from build123d import *

# Parameters (mm, degrees)
EXTRUDE_1_DEPTH        = 6
HOLE_WIZARD_M6_1_D     = 5
HOLE_WIZARD_M6_1_DEPTH = 18
HOLE_WIZARD_M6_1_TIP   = 1.502151548
FILLET_1_R             = 10
HOLE_WIZARD_M10_1_D    = 8.5


with BuildPart() as part:
    # 草图1 → 凸台-拉伸1 (new body, symmetric)
    with BuildSketch(Plane.XY):
        Polygon((0, 0), (75, 0), (75, 15), (120, 15), (120, 40), (0, 40), align=None)
    extrude(amount=EXTRUDE_1_DEPTH, both=True)

    # M6 螺纹孔1
    with Locations(Plane(origin=(0, 0, 0), x_dir=(-1, 0, 0), z_dir=(0, -1, 0))):
        with Locations((-10, 0), (-65, 0)):
            Hole(HOLE_WIZARD_M6_1_D / 2, depth=HOLE_WIZARD_M6_1_DEPTH)
            with Locations((0, 0, -(HOLE_WIZARD_M6_1_DEPTH + HOLE_WIZARD_M6_1_TIP / 2))):  # 118° drill point
                Cone(0, HOLE_WIZARD_M6_1_D / 2, HOLE_WIZARD_M6_1_TIP, mode=Mode.SUBTRACT)

    # 圆角1
    fillet_1_edges = [part.edges().sort_by_distance(p)[0] for p in [
        (0, 40, 0),
        (120, 40, 0),
        (120, 15, 0),
        (75, 15, 0),
    ]]
    fillet(fillet_1_edges, radius=FILLET_1_R)

    # M10 螺纹孔1 (through all)
    with Locations(Plane.XY.offset(6)):
        with Locations((105, 28)):
            Hole(HOLE_WIZARD_M10_1_D / 2)


solid = part.part
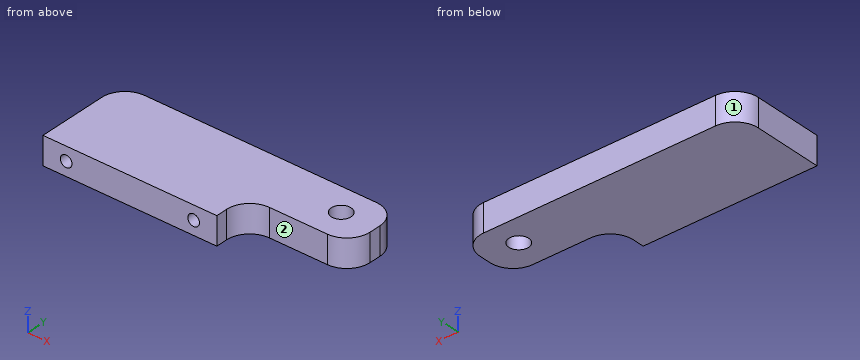
Verification items for the finished model (mm, model axes). Face numbers are marked on the shaded views. A direction names the side the tool comes from. Coordinates: 2 decimals unless noted, no trailing zeros. Loops run counter-clockwise (first coordinate to the right, second up) from the corner with the lowest first, then second, coordinate; pieces in that order, holes last. Notation, with made-up numbers: M -18.5,3.25 L -2.5,3.25 A28 ccw -2.5,41.25 Z; hole C 1,43.25 d5. An arc over 180 degrees is marked long. One line per item, written item: value.
1. Section check B-B on z = -4.25. Record the cut outline in (x, y), plus the area to 3 significant figures.
Answers follow:
outline: M 0,0 L 75,0 L 75,5 A10 cw 85,15 L 110,15 A10 ccw 120,25 L 120,30 A10 ccw 110,40 L 10,40 A10 ccw 0,30 Z; hole C 105,28 d8.5
area: 4,030 mm^2
2. Gauge pin test, flat ends, axial feed: P1, Ø4, axis at x = 65, z = 0, coming from the -Y side; P2, Ø3.5, axis at x = 103, z = 0, coming from the -Y side; P3, Ø5.5, axis at y = 3, z = 0.5, coming from the +X side. Record the tip position at first contact, or that the pin passes through.
Answers follow:
P1: y = 18.3
P2: y = 15
P3: x = 75.03
3. Section check A-A on y = 28. Record the cut outline in (x, z), plus the area to 3 significant figures.
Answers follow:
outline: M 0,-6 L 100.75,-6 L 100.75,6 L 0,6 Z; M 109.25,-6 L 120,-6 L 120,6 L 109.25,6 Z
area: 1,340 mm^2
4. Material ranges on line 1 along Z through (x, y) = (65, 11); line 2 along Y through (x, z) = (105, -1.5); line 3 along X through (y, z) = (3.5, 3.25), recorded low to high. Write a range as from..to.
Answers follow:
line 1: -6..-2.5, 2.5..6
line 2: 15..23.75, 32.25..40
line 3: 0..75
5. Section check C-C on x = 104. Record the cut outline in (y, z).
Answers follow:
outline: M 15,-6 L 23.87,-6 L 23.87,6 L 15,6 Z; M 32.13,-6 L 40,-6 L 40,6 L 32.13,6 Z
6. Set-up check for the marked faces 1 and 2: record each of +Z, -Z, +X, -X, +Y, -Y from which the full face is reachable in a straight line by a thin tool's end or side.
Answers follow:
face 1: +Z, -Z, -X, +Y
face 2: +Z, -Z, +X, -Y
7. Section check D-D on x = 90.5. Record the cut outline in (y, z), plus the area to 3 significant figures.
Answers follow:
outline: M 15,-6 L 40,-6 L 40,6 L 15,6 Z
area: 300 mm^2
